Autodesk Inventor part; units mm, degrees
ref_plane "MidSidePlane" through (0, 0, 10) normal (0, 0, 1) x (1, 0, 0)
ref_plane "YZ Plane" through (0, 0, 0) normal (1, 0, 0) x (0, 1, 0)
ref_plane "XZ Plane" through (0, 0, 0) normal (0, 1, 0) x (-1, 0, 0)
sketch "ShaftProfile" plane through (0, 0, 0) normal (0, 0, 1) x (1, 0, 0)
  line L0 (-52, 0) -> (46, 0) construction
  line L1 (-38, 9) -> (32, 9)
  line L2 (32, 9) -> (32, 0)
  line L3 (-38, 0) -> (-38, 9)
  line L4 (-38, 0) -> (32, 0)
  point P0 (0, 0)
  dimension "d1" = 70
  dimension "d2" = 9
  dimension "d4" = 38
revolve "ShaftFeature" add sketch "ShaftProfile" angle 360 about axis through (-38, 0, 0) along (1, 0, 0)
sketch "Sketch2" plane through (-38, 0, 0) normal (-1, 0, 0) x (0, 0, 1)
  circle A0 centre (0, 0) radius 9
hole "ShaftHoleFeature" at (-38, 0, 0) direction (1, 0, 0) diameter 16 end through all
ref_plane "MidSidePlane" through (0, 0, 10) normal (0, 0, 1) x (1, 0, 0)
sketch "CapHoles" plane through (0, 0, 10) normal (0, 0, 1) x (1, 0, 0)
  line L0 (32, -9) -> (32, 9) construction
  line L1 (-38, -9) -> (-38, 9) construction
  line L2 (-53, 0) -> (52, 0) construction
  circle A0 centre (-33.5, 0) radius 1.25
  circle A1 centre (27.5, 0) radius 1.25
  dimension "d24" = 2.5
  dimension "d25" = 4.5
  dimension "d26" = 4.5
extrude "CapHolesFeature" cut sketch "CapHoles" against normal through all
equation "\"d26\" = d25"
properties part number "BackPair1PistonShaft"
Input: part model. Units: mm. Frame: model coordinates. Coordinates: 2 decimals unless noted, no trailing zeros. Loops run counter-clockwise (first coordinate to the right, second up) from the corner with the lowest first, then second, coordinate; pieces in that order, holes last.
(1) Material intervals for probe 1 along X at (y, z) = (0, 8.4); probe 2 along Z at (x, y) = (-10, 0.5); probe 3 along Y at (x, z) = (27.5, 8.2), sorted ascending.
(2) Section D-D on x = -10. Return the cut outline in (y, z).
(3) Pull-direction query (X, two-part tool) for faces 1 (the face through (28.172, 1.054, -8.443)), 2 (the face through (26.25, 0.05, 8.46)); classes: released by +X, released by -X, zero draft, split by the parting line, or undercut.
(4) First-contact query: pin 1 Ø4 at (y, z) = (3.5, 2.5) entering from +X; pin 2 Ø1 at (x, z) = (-15, -3) entering from +Y; pin 3 Ø6 at (x, y) = (-20.5, -4) entering from -Z; pin 4 Ø5 at (x, y) = (-23, 5.5) entering from +Z. Flat tips, straight axial feed; report the tip coordinate or a pass-through.
(5) Section B-B on y = 0. Return the cut outline in (x, z), then the cut area to 3 significant figures.
(6) Section C-C on x = -33.5. Return the cut outline in (y, z), then the cut area to 3 significant figures.
(7) Section A-A on z = 0. Return the cut outline in (x, y), then the cut area to 3 significant figures.
Data:
1. probe 1: x = -38 to -34.75, -32.25 to 26.25, 28.75 to 32
1. probe 2: z = -8.99 to -7.98, 7.98 to 8.99
1. probe 3: y = -3.71 to -1.25, 1.25 to 3.71
2. outline: circle Ø18 at (0, 0); hole circle Ø16 at (0, 0)
3. face 1: undercut
3. face 2: undercut
4. pin 1: passes through
4. pin 2: stops at y = 8.65
4. pin 3: stops at z = -8.94
4. pin 4: stops at z = 8.49
5. outline: (-38, -9) - (-34.75, -9) - (-34.75, -8) - (-38, -8) - close; (-38, 8) - (-34.75, 8) - (-34.75, 9) - (-38, 9) - close; (-32.25, -9) - (26.25, -9) - (26.25, -8) - (-32.25, -8) - close; (-32.25, 8) - (26.25, 8) - (26.25, 9) - (-32.25, 9) - close; (28.75, -9) - (32, -9) - (32, -8) - (28.75, -8) - close; (28.75, 8) - (32, 8) - (32, 9) - (28.75, 9) - close
5. area: 130 mm2
6. outline: (-1.25, -8.91) - (-1.25, -7.9) arc R8 cw to (-1.25, 7.9) - (-1.25, 8.91) arc R9 ccw to start; (1.25, -8.91) arc R9 ccw to (1.25, 8.91) - (1.25, 7.9) arc R8 cw to (1.25, -7.9) - close
6. area: 48.4 mm2
7. outline: (-38, -9) - (32, -9) - (32, -8) - (-38, -8) - close; (-38, 8) - (32, 8) - (32, 9) - (-38, 9) - close
7. area: 140 mm2
